Autodesk Inventor part; units mm, degrees
ref_plane "YZ Plane" through (0, 0, 0) normal (1, 0, 0) x (0, 1, 0)
ref_plane "XZ Plane" through (0, 0, 0) normal (0, 1, 0) x (-1, 0, 0)
ref_plane "XY Plane" through (0, 0, 0) normal (0, 0, 1) x (1, 0, 0)
sketch "Sketch1" plane through (0, 0, 0) normal (1, 0, 0) x (0, 1, 0)
  line L0 (28.3233, 27.0734) -> (-24.0767, 27.0734)
  line L1 (-26.0767, 25.0734) -> (-26.0767, -27.3266)
  line L2 (-24.0767, -29.3266) -> (28.3233, -29.3266)
  line L3 (30.3233, -27.3266) -> (30.3233, 25.0734)
  arc A0 (-24.0767, 27.0734) -> (-26.0767, 25.0734) centre (-24.0767, 25.0734) ccw
  arc A1 (30.3233, 25.0734) -> (28.3233, 27.0734) centre (28.3233, 25.0734) ccw
  arc A2 (28.3233, -29.3266) -> (30.3233, -27.3266) centre (28.3233, -27.3266) ccw
  arc A3 (-26.0767, -27.3266) -> (-24.0767, -29.3266) centre (-24.0767, -27.3266) ccw
  point P0 (0, 0)
  point P1 (30.3233, 27.0734)
  point P2 (-26.0767, -29.3266)
  point P3 (-26.0767, 27.0734)
  point P4 (30.3233, -29.3266)
  dimension "d0" = 56.4
  dimension "d1" = 56.4
  dimension "d18" = 2
extrude "Extrusion1" add sketch "Sketch1" along normal blind 16
sketch "Sketch5" plane through (16, 0, 0) normal (1, 0, 0) x (0, 0, -1)
  circle A0 centre (24.6966, 25.6933) radius 2.5
  circle A1 centre (24.6966, -21.4467) radius 2.5
  circle A2 centre (-22.4434, -21.4467) radius 2.5
  circle A3 centre (-22.4434, 25.6933) radius 2.5
  point P0 (0, 0)
  dimension "d38" = 5
  dimension "d39" = 5
  dimension "d40" = 5
  dimension "d41" = 5
extrude "Extrusion3" cut sketch "Sketch5" against normal blind 16
sketch "Sketch6" plane through (16, 0, 0) normal (1, 0, 0) x (0, 0, -1)
  line L0 (-25.0734, -26.0767) -> (27.3266, -26.0767)
  arc A0 (27.3266, -26.0767) -> (29.3266, -24.0767) centre (27.3266, -24.0767) ccw
  circle A1 centre (-22.4434, -21.4467) radius 2.5
  circle A2 centre (24.6966, 25.6933) radius 2.5
  circle A3 centre (24.6966, -21.4467) radius 2.5
  circle A4 centre (-22.4434, 25.6933) radius 2.5
  line L1 (-27.0734, 28.3233) -> (-27.0734, -24.0767)
  arc A5 (-27.0734, -24.0767) -> (-25.0734, -26.0767) centre (-25.0734, -24.0767) ccw
  line L2 (-25.0734, -26.0767) -> (27.3266, -26.0767)
  arc A6 (27.3266, -26.0767) -> (29.3266, -24.0767) centre (27.3266, -24.0767) ccw
  line L3 (29.3266, -24.0767) -> (29.3266, 28.3233)
  arc A7 (29.3266, 28.3233) -> (27.3266, 30.3233) centre (27.3266, 28.3233) ccw
  line L4 (27.3266, 30.3233) -> (-25.0734, 30.3233)
  arc A8 (-25.0734, 30.3233) -> (-27.0734, 28.3233) centre (-25.0734, 28.3233) ccw
  line L5 (20.0666, 30.3233) -> (20.0666, 21.0633)
  line L6 (20.0666, 21.0633) -> (29.3266, 21.0633)
  line L7 (20.0666, -26.0767) -> (20.0666, -16.8167)
  line L8 (20.0666, -16.8167) -> (29.3266, -16.8167)
  line L9 (-17.8134, 30.3233) -> (-17.8134, 21.0633)
  line L10 (-17.8134, 21.0633) -> (-27.0734, 21.0633)
  line L11 (-17.8134, -26.0767) -> (-17.8134, -16.8167)
  line L12 (-17.8134, -16.8167) -> (-27.0734, -16.8167)
  line L13 (29.3266, 21.0633) -> (29.3266, -16.8167)
  line L14 (20.0666, 30.3233) -> (-17.8134, 30.3233)
  line L15 (-25.0734, 30.3233) -> (27.3266, 30.3233)
  line L16 (-27.0734, 21.0633) -> (-27.0734, -16.8167)
  line L17 (-27.0734, -24.0767) -> (-27.0734, 28.3233)
  line L18 (20.0666, -26.0767) -> (-17.8134, -26.0767)
  line L19 (27.3266, -26.0767) -> (-25.0734, -26.0767)
  point P0 (0, 0)
  dimension "d44" = 9.26
  dimension "d45" = 9.26
  dimension "d46" = 9.26
  dimension "d47" = 9.26
  dimension "d48" = 9.26
  dimension "d49" = 9.26
  dimension "d50" = 9.26
  dimension "d51" = 9.26
extrude "Extrusion4" add sketch "Sketch6" along normal blind 55 contours L11 L12 L1 L10 L9 L4 L5 L6 L3 L8 L7 L0
sketch "Sketch7" plane through (71, 0, 0) normal (1, 0, 0) x (0, 0, -1)
  line L0 (27.3266, -26.0767) -> (-25.0734, -26.0767)
  line L1 (-27.0734, -24.0767) -> (-27.0734, 28.3233)
  line L2 (-25.0734, 30.3233) -> (27.3266, 30.3233)
  line L3 (29.3266, 28.3233) -> (29.3266, -24.0767)
  arc A0 (27.3266, -26.0767) -> (29.3266, -24.0767) centre (27.3266, -24.0767) ccw
  arc A1 (-27.0734, -24.0767) -> (-25.0734, -26.0767) centre (-25.0734, -24.0767) ccw
  arc A2 (-25.0734, 30.3233) -> (-27.0734, 28.3233) centre (-25.0734, 28.3233) ccw
  arc A3 (29.3266, 28.3233) -> (27.3266, 30.3233) centre (27.3266, 28.3233) ccw
  point P0 (0, 0)
  point P1 (-27.0734, 30.3233)
  point P2 (-27.0734, -26.0767)
  point P3 (29.3266, 30.3233)
  dimension "d54" = 56.4
  dimension "d55" = 56.4
  dimension "d56" = 2
extrude "Extrusion5" add sketch "Sketch7" along normal blind 5
fillet "Fillet1" radius 2 12 edges at (43.5, -16.8167, -29.3266) (43.5, -16.8167, -20.0666) (43.5, -26.0767, -20.0666) (43.5, -16.8167, 27.0734) (43.5, -16.8167, 17.8134) (43.5, -26.0767, 17.8134) (43.5, 21.0633, 27.0734) (43.5, 21.0633, 17.8134) (43.5, 30.3233, 17.8134) (43.5, 30.3233, -20.0666) (43.5, 21.0633, -20.0666) (43.5, 21.0633, -29.3266)
sketch "Sketch8" plane through (0, 0, 0) normal (-1, 0, 0) x (0, 0, 1)
  line L0 (-29.3266, 28.3233) -> (-29.3266, -24.0767)
  line L1 (-27.3266, -26.0767) -> (25.0734, -26.0767)
  line L2 (27.0734, -24.0767) -> (27.0734, 28.3233)
  line L3 (25.0734, 30.3233) -> (-27.3266, 30.3233)
  arc A0 (-27.3266, 30.3233) -> (-29.3266, 28.3233) centre (-27.3266, 28.3233) ccw
  arc A1 (27.0734, 28.3233) -> (25.0734, 30.3233) centre (25.0734, 28.3233) ccw
  arc A2 (25.0734, -26.0767) -> (27.0734, -24.0767) centre (25.0734, -24.0767) ccw
  circle A3 centre (-1.1266, 2.1233) radius 0.0027
  circle A4 centre (-1.1266, 2.1233) radius 19.05
  point P0 (0, 0)
  dimension "d60" = 38.1
extrude "Extrusion6" add sketch "Sketch8" along normal blind 1.6
sketch "Sketch9" plane through (-1.6, 2.1233, -1.1266) normal (-1, 0, 0) x (0, 0, 1)
  circle A0 centre (0, 0) radius 3.175
  point P0 (1.1266, -2.1233)
  dimension "d63" = 6.35
extrude "Extrusion7" add sketch "Sketch9" along normal blind 20.6
sketch "Sketch10" plane through (0, 0, 0) normal (-1, 0, 0) x (0, 0, 1)
  point P0 (0, 0)
properties part number "MOTOR"
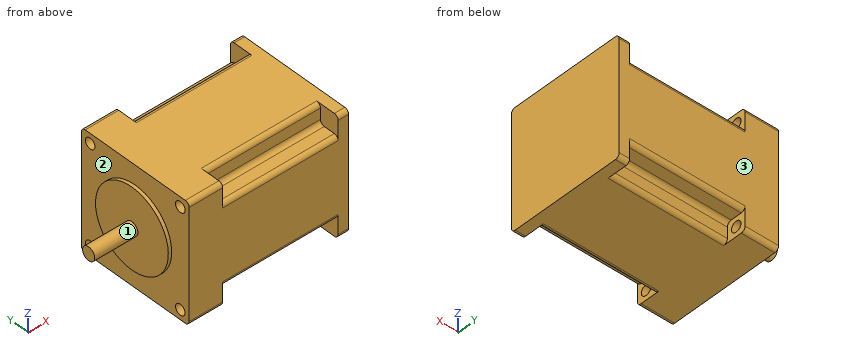
Verification items for the finished model (mm, model axes). Face numbers are marked on the shaded views. Coordinates: 2 decimals unless noted, no trailing zeros. Order: outer loops, then holes, each group sorted by start corner. A loop starts at its lowest first (then second) coordinate and runs counter-clockwise, first axis right, second up. Notation, with made-up numbers: (51, 77) -> (99, 77) arc R11 ccw to (99, 81) -> close; hole circle Ø8 at (16, -19). An arc over 180 degrees is marked (long way). Put each result on its own line as item: value. Start each with the question number.
1. Go/stop test with flat-tipped pins: pin 1 Ø1.6 at (x, z) = (42, -24.5) entering from -Y; pin 2 Ø3.5 at (y, z) = (-19.5, -22.5) entering from -X; pin 3 Ø1.6 at (x, y) = (43, 26) entering from +Z. Record where each tip stops, or that it passes through.
2. Cross-section at B-B, the plane z = 23.5. Record the boundary of the cut face in (x, y), then the cut area to 3 significant figures.
3. Cross-section at C-C, the plane x = 5. Record the boundary of the cut face in (y, z).
4. Cross-section at D-D, the plane y = 10.5. Record the boundary of the cut face in (x, z), then the cut area to 3 significant figures.
5. Mould release check, pull along Y, two halves, no side actions. Record for the marked faces 1, 2 and 3: released by +Y, released by -Y, zero draft, split by the parting line, or undercut.
6. Cross-section at A-A, the plane x = 62. Record the boundary of the cut face in (y, z).
7. Material ranges on L1, parallel to X at y = -19, z = 19.5; L2, parallel to Z at x = 69, y = 24; L3, parallel to X at y = 6.5, z = 14, recorded low to high. Write a range as [from, to].
Computed:
1. pin 1: y = -16.82
1. pin 2: x = 0
1. pin 3: z = 17.81
2. outline: (0, -26.08) -> (16, -26.08) -> (16, -23.71) -> (0, -23.71) -> close; (0, -19.18) -> (16, -19.18) -> (16, -16.82) -> (71, -16.82) -> (71, -26.08) -> (76, -26.08) -> (76, 30.32) -> (71, 30.32) -> (71, 21.06) -> (16, 21.06) -> (16, 23.43) -> (0, 23.43) -> close; (0, 27.96) -> (16, 27.96) -> (16, 30.32) -> (0, 30.32) -> close
2. area: 3,120 mm2
3. outline: (-26.08, -27.33) arc R2 ccw to (-24.08, -29.33) -> (28.32, -29.33) arc R2 ccw to (30.32, -27.33) -> (30.32, 25.07) arc R2 ccw to (28.32, 27.07) -> (-24.08, 27.07) arc R2 ccw to (-26.08, 25.07) -> close; hole circle Ø5 at (-21.45, -24.7); hole circle Ø5 at (-21.45, 22.44); hole circle Ø5 at (25.69, -24.7); hole circle Ø5 at (25.69, 22.44)
4. outline: (-1.6, -18.24) -> (0, -18.24) -> (0, -29.33) -> (76, -29.33) -> (76, 27.07) -> (0, 27.07) -> (0, 15.98) -> (-1.6, 15.98) -> close
4. area: 4,340 mm2
5. face 1: split by the parting line
5. face 2: zero draft
5. face 3: released by +Y
6. outline: (-26.08, -18.07) arc R2 ccw to (-24.08, -20.07) -> (-18.82, -20.07) arc R2 cw to (-16.82, -22.07) -> (-16.82, -27.33) arc R2 ccw to (-14.82, -29.33) -> (19.06, -29.33) arc R2 ccw to (21.06, -27.33) -> (21.06, -22.07) arc R2 cw to (23.06, -20.07) -> (28.32, -20.07) arc R2 ccw to (30.32, -18.07) -> (30.32, 15.81) arc R2 ccw to (28.32, 17.81) -> (23.06, 17.81) arc R2 cw to (21.06, 19.81) -> (21.06, 25.07) arc R2 ccw to (19.06, 27.07) -> (-14.82, 27.07) arc R2 ccw to (-16.82, 25.07) -> (-16.82, 19.81) arc R2 cw to (-18.82, 17.81) -> (-24.08, 17.81) arc R2 ccw to (-26.08, 15.81) -> close
7. L1: [0, 16], [71, 76]
7. L2: [-20.07, 17.81]
7. L3: [-1.6, 76]
